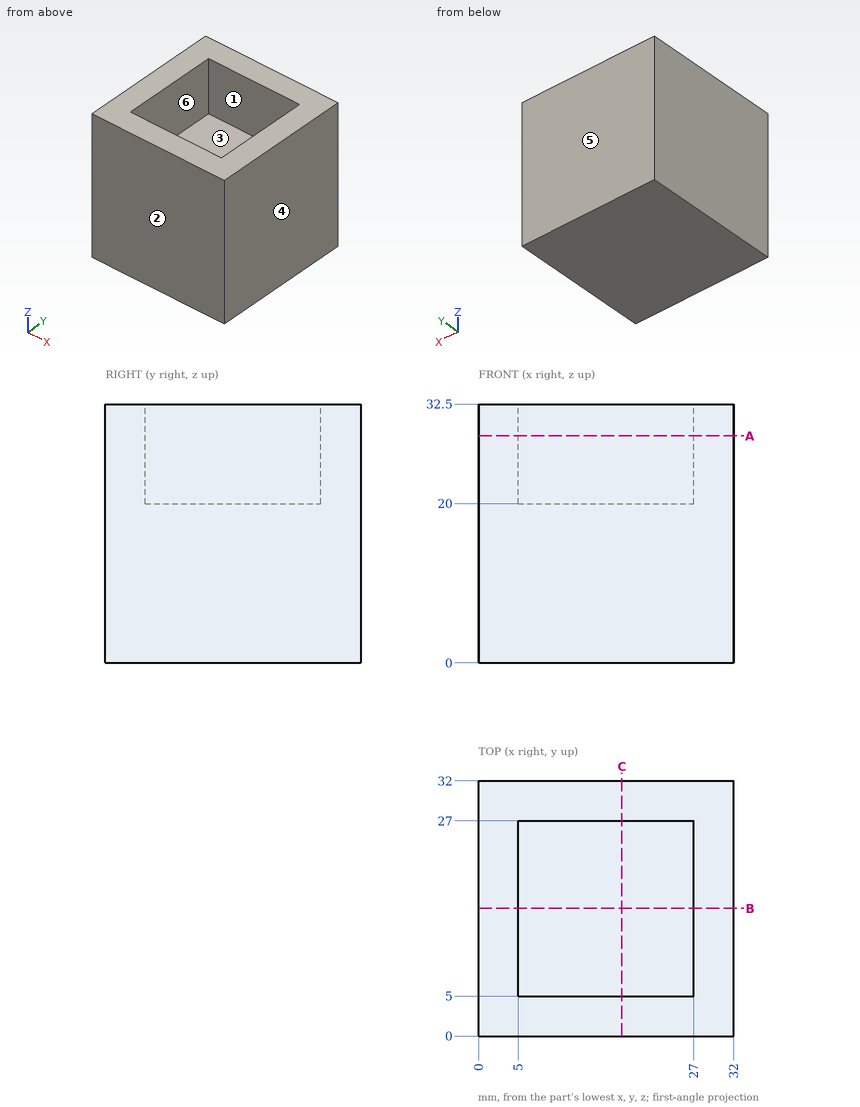
Source: three-view drawing plus pictorial views. Frame: mm from the lowest corner of the part. A direction names the side the tool comes from. Give positions to 0.01 mm unless a question says otherwise; leave off trailing zeros. Write each loop counter-clockwise with the first axis right and the second up, starting at its lowest first coordinate (ties: lowest second). Pieces come first, ordered by that corner, then holes. Notation, with made-up numbers: (38, 54) -> (89, 54) arc R24 cw to (89, 85) -> close; hole circle Ø1 at (-7.5, 35.5). An arc over 180 degrees is marked (long way). Write item = value, one per line.
Q1. First-contact query: pin 1 (4 mm diameter, centred on x = 14, y = 11, fed in from +Z). Flat tip, straight axial feed; report the tip coordinate or a pass-through.
Here are the results:
pin_1 = 20
Q2. Mould query, pull axis Y, two halves, no side actions, for the marked faces 3, 4, 5 and 6. Classes: +Y half, -Y half, draft (parallel to the pull), parting line (faces both ways), or undercut.
Here are the results:
face_3 = undercut
face_4 = draft
face_5 = +Y half
face_6 = undercut
Q3. Line query: line 1 (Y direction, x = 16.5, z = 25); line 2 (Z direction, x = 25, y = 22). Output: solid intervals per line, ascending. Write a range as from..to.
Here are the results:
line_1 = 0..5, 27..32
line_2 = 0..20
Q4. Cut plane A-A on z = 28.5. Return loops of the section in (x, y).
Here are the results:
outline = (0, 0) -> (32, 0) -> (32, 32) -> (0, 32) -> close; hole (5, 5) -> (27, 5) -> (27, 27) -> (5, 27) -> close
Q5. Reachability of the marked faces 1 and 2 from +Z, -Z, +X, -X, +Y, -Y: full face, straight path, thin tool, end or side. Return the list, or none.
Here are the results:
face_1 = +Z
face_2 = +Z, -Z, +X, -X, -Y
Q6. Cut plane B-B on y = 16. Return loops of the section in (x, z).
Here are the results:
outline = (0, 0) -> (32, 0) -> (32, 32.5) -> (27, 32.5) -> (27, 20) -> (5, 20) -> (5, 32.5) -> (0, 32.5) -> close
